Check sheet for the modelled part. Datum: model origin and axes. Units: mm. Coordinates: 2 decimals unless noted, no trailing zeros. Loops run counter-clockwise (first coordinate to the right, second up) from the corner with the lowest first, then second, coordinate; pieces in that order, holes last. Notation, with made-up numbers: (41.5, -35.5) - (78.5, -35.5) arc R7 ccw to (78.5, -22.5) - close; hole circle Ø3 at (14, 16.5). An arc over 180 degrees is marked (long way). Answer as a JSON object with one key per item and string values. Group by question number.
from build123d import *

# Parameters (mm, degrees)
F1_DEPTH = 6
F2_SIZE  = 5.99999
F3_R     = 1.5
F4_DEPTH = 6


# Not quite as in the source:
# - a fillet or chamfer is up to 0.001 mm smaller than in the source, because OpenCascade refuses the exact size


with BuildPart() as f1:
    # F0 (on Top) → F1 (new body)
    with BuildSketch(Plane.XY):
        Polygon((10.2662842423, 7.4127185345), (-3.7337157577, 7.4127185345), (-3.7337157577, -10.0872814655), (10.2662842423, -13.5872814655), align=None)
    extrude(amount=F1_DEPTH)

    # F2 (size 6 in the source; OpenCascade refuses exactly that, so slightly less here)
    f2_edges = [f1.edges().sort_by_distance(p)[0] for p in [
        (3.266284, -11.837281, 0),
    ]]
    chamfer(f2_edges, length=F2_SIZE)

    # F3 (on face) → F4 (cut, through all)
    with BuildSketch(Plane.XY.offset(6)):
        with Locations((-1.7337157577, 1.4127185345)):
            Circle(F3_R)
        with Locations((8.2662842423, 1.4127185345)):
            Circle(F3_R)
    extrude(amount=-F4_DEPTH, mode=Mode.SUBTRACT)


solid = f1.part
1. Sectioned sample at D-D on y = -6.5. Record the cut outline in (x, z).
2. Material ranges on line 1 (X direction, y = 1.5, z = 5.5); line 2 (Y direction, x = 9.25, z = 4); line 3 (X direction, y = 2.75, z = 4), recorded low to high.
3. Release check for a two-part mould opening along Y. For faces 1 (the face through (-0.3, 1.86, 3.04)), 2 (the face through (7.161, 2.426, 3.042)), 3 (the face through (3, 7.413, 3)), 4 (the face through (3, 0, 0)) record: released by +Y, released by -Y, zero draft, split by the parting line, or undercut.
4. Sectioned sample at B-B on z = 4. Record the cut outline in (x, y).
5. Gauge pin test, flat ends, axial feed: pin 1 (2.5 mm diameter, centred on x = 8.27, y = 1.41, fed in from -Z); pin 2 (1.5 mm diameter, centred on x = 4, z = 1, fed in from -Y); pin 3 (6 mm diameter, centred on x = 2, y = -9.5, fed in from -Z). Record the tip position at first contact, or that the pin passes through.
Answers follow:
{
 "1": {"outline": "(-3.73, 2.52) - (6.66, 0) - (10.27, 0) - (10.27, 6) - (-3.73, 6) - close"},
 "2": {"line 1": "x = -3.73 to -3.23, -0.24 to 6.77, 9.76 to 10.27", "line 2": "y = -11.27 to 0.28, 2.55 to 7.41", "line 3": "x = -3.73 to -2.41, -1.05 to 7.59, 8.95 to 10.27"},
 "3": {"face 1": "undercut", "face 2": "undercut", "face 3": "released by +Y", "face 4": "zero draft"},
 "4": {"outline": "(-3.73, -8.03) - (10.27, -11.53) - (10.27, 7.41) - (-3.73, 7.41) - close; hole circle Ø3 at (-1.73, 1.41); hole circle Ø3 at (8.27, 1.41)"},
 "5": {"pin 1": "passes through", "pin 2": "stops at y = -7.66", "pin 3": "stops at z = 1.04"}
}
